```python
from build123d import *

# Parameters (mm, degrees)
SKETCH1_R           = 3
BOSS_EXTRUDE1_DEPTH = 5
SKETCH2_W           = 14.277681963
SKETCH2_H           = 5.610279578
CUT_EXTRUDE1_DEPTH  = 3
BOSS_EXTRUDE2_DEPTH = 6
CHAMFER1_SIZE       = 3
CHAMFER1_SIZE2      = 4


with BuildPart() as part:
    # Sketch1 → Boss-Extrude1 (new body)
    with BuildSketch(Plane.XY):
        with BuildLine():
            Line((0, 0), (7, 0))
            Line((7, 0), (7, 9))
            Line((7, 9), (4, 9))
            Line((4, 9), (4, 10))
            Line((4, 10), (0, 10))
            ThreePointArc((0, 10), (-5, 5), (0, 0))
        make_face()
        with Locations((0, 5)):
            Circle(SKETCH1_R, mode=Mode.SUBTRACT)
    extrude(amount=BOSS_EXTRUDE1_DEPTH)

    # Sketch2 → Cut-Extrude1 (cut)
    with BuildSketch(Plane.XY.offset(5)):
        with Locations((2.138840982, 7.805139789)):
            Rectangle(SKETCH2_W, SKETCH2_H)
    extrude(amount=-CUT_EXTRUDE1_DEPTH, mode=Mode.SUBTRACT)

    # Sketch3 → Boss-Extrude2 (add)
    with BuildSketch(Plane.XY.offset(2)):
        Polygon((7, 7), (6, 7), (3, 1), (3, 0), (7, 0), align=None)
    extrude(amount=BOSS_EXTRUDE2_DEPTH)

    # Chamfer1
    chamfer1_edges = [part.edges().sort_by_distance(p)[0] for p in [
        (6.5, 7, 8),
    ]]
    chamfer1_side = [part.faces().sort_by_distance(p)[0] for p in [
        (6.5, 7, 5),
    ]]
    chamfer(chamfer1_edges, length=CHAMFER1_SIZE, length2=CHAMFER1_SIZE2, reference=chamfer1_side[0])


solid = part.part
```
CAD build for the part. Positions are in the model's coordinates, mm. A direction names the side the tool comes from. Give positions to 0.01 mm unless a question says otherwise; leave off trailing zeros. Loops run counter-clockwise (first coordinate to the right, second up) from the corner with the lowest first, then second, coordinate; pieces in that order, holes last. Notation, with made-up numbers: (8.25, 19) -> (60.25, 19) arc R26 ccw to (60.25, 53) -> close; hole circle Ø5 at (48, 66). An arc over 180 degrees is marked (long way). Use a Markdown table: item, result.
1. Which spindle directions (+Z, -Z, +X, -X, +Y, -Y) get a long thin tool onto all of the face, cutting with end or side? Do faces 1 (the flat face through (7, 3, 3)), 2 (the flat face through (6, 9, 1)), 3 (the flat face through (3, 0.5, 6.5)), 4 (the flat face through (1, 8, 2)), 5 (the flat face through (6.5, 7, 3.5)). Say none if no direction does.
Check result:
| item | result |
|---|---|
| face 1 | +Z, -Z, +X, +Y, -Y |
| face 2 | +Z, -Z, +X, +Y |
| face 3 | +Z, -X, +Y, -Y |
| face 4 | +Z, -X, +Y |
| face 5 | +Z, +X, -X, +Y |
2. Slice it at C-C (x = -2). List the corners of the cut face in (y, z).
Check result:
| item | result |
|---|---|
| outline | (0.42, 0) -> (2.76, 0) -> (2.76, 5) -> (0.42, 5) -> close; (7.24, 0) -> (9.58, 0) -> (9.58, 2) -> (7.24, 2) -> close |
3. Wall check: L1, parallel to Z at x = -3.75, y = 3; L2, parallel to Y at x = 0, z = 2.55; L3, parallel to X at y = 5, z = 1.4. Give the ranges that are in metal, low to high. Write a range as [from, to].
Check result:
| item | result |
|---|---|
| L1 | z = [0, 5] |
| L2 | y = [0, 2] |
| L3 | x = [-5, -3], [3, 7] |
4. Slice it at B-B (y = 4.5). List the corners of the cut face in (x, z) (3 decimals), plus the area to 3 significant figures.
Check result:
| item | result |
|---|---|
| outline | (-4.975, 0) -> (-2.958, 0) -> (-2.958, 5) -> (-4.975, 5) -> close; (2.958, 0) -> (7, 0) -> (7, 6.875) -> (4.75, 6.875) -> (4.75, 5) -> (2.958, 5) -> close |
| area | 34.5 mm^2 |
5. Slice it at A-A (z = 2.5). List the corners of the cut face in (x, y).
Check result:
| item | result |
|---|---|
| outline | (-5, 5) arc R5 ccw to (0, 0) -> (7, 0) -> (7, 7) -> (6, 7) -> (5, 5) -> (3, 5) arc R3 cw to (-3, 5) -> close |
6. Flat gauge pins, fed straight in: pin 1 (1.1 mm diameter, centred on x = 6.5, z = 3.5, fed in from +Y); pin 2 (0.8 mm diameter, centred on y = 9.5, z = 1.5, fed in from +X); pin 3 (1.6 mm diameter, centred on x = 3.5, z = 3.5, fed in from +Y). Where does each tip first touch, or does it go through?
Check result:
| item | result |
|---|---|
| pin 1 | stops at y = 7 |
| pin 2 | stops at x = 4 |
| pin 3 | stops at y = 5 |
7. Slice it at D-D (x = 3.5). List the corners of the cut face in (y, z).
Check result:
| item | result |
|---|---|
| outline | (0, 0) -> (10, 0) -> (10, 2) -> (5, 2) -> (5, 5) -> (2, 5) -> (2, 8) -> (0, 8) -> close |
8. Mould opens along X. For faces 6 (the flat face through (-1, 2, 5)), 7 (the flat face through (4, 9.5, 1)), 8 (the cylindrical face through (-0.65, 2.07, 1.91)) say: pulls with the +X half, pulls with the -X half, needs draft (parallel to the pull), parting line crosses it, or undercut.
Check result:
| item | result |
|---|---|
| face 6 | needs draft |
| face 7 | pulls with the +X half |
| face 8 | undercut |
